from build123d import *

# Parameters (mm, degrees)
SKETCH1_R           = 3
SKETCH1_R_2         = 0.5
BOSS_EXTRUDE1_DEPTH = 5
CUT_EXTRUDE1_DEPTH  = 25
CUT_EXTRUDE2_DEPTH  = 2
SKETCH4_W           = 1
SKETCH4_H           = 3
CUT_EXTRUDE3_DEPTH  = 3


with BuildPart() as part:
    # Sketch1 → Boss-Extrude1 (new body)
    with BuildSketch(Plane.XY):
        with BuildLine():
            Line((-9.495764101, 3), (-6.495764101, 5))
            Line((-6.495764101, 5), (5.504235899, 5))
            ThreePointArc((5.504235899, 5), (9.046847958, 3.528441554), (10.504195739, -0.02004008))
            ThreePointArc((10.504195739, -0.02004008), (9.032677453, -3.542612059), (5.504235899, -5))
            Line((5.504235899, -5), (-6.495764101, -5))
            Line((-6.495764101, -5), (-9.495764101, -3))
            Line((-9.495764101, -3), (-9.495764101, 3))
        make_face()
        with Locations((-4.495764101, 0)):
            Circle(SKETCH1_R, mode=Mode.SUBTRACT)
        with Locations((-0.495764101, 0)):
            Circle(SKETCH1_R_2, mode=Mode.SUBTRACT)
        with BuildLine():
            Line((2.504235899, 2), (5.504235899, 2))
            ThreePointArc((5.504235899, 2), (7.504235899, 0), (5.504235899, -2))
            Line((5.504235899, -2), (2.504235899, -2))
            ThreePointArc((2.504235899, -2), (0.504235899, 0), (2.504235899, 2))
        make_face(mode=Mode.SUBTRACT)
    extrude(amount=BOSS_EXTRUDE1_DEPTH)

    # Sketch2 → Cut-Extrude1 (cut)
    with BuildSketch(Plane(origin=(0, 5, 0), x_dir=(1, 0, 0), z_dir=(0, 1, 0))):
        Polygon((-9.495764101, -2), (-2.495764101, -2), (-2.495764101, -3), (4.450061274, -3), (4.450061274, -5), (9.504235899, -5), (9.504235899, -3), (10.504235899, -3), (10.504235899, -6.643116644), (-9.495764101, -6.643116644), align=None)
    extrude(amount=-CUT_EXTRUDE1_DEPTH, mode=Mode.SUBTRACT)

    # Sketch3 → Cut-Extrude2 (cut)
    with BuildSketch(Plane.XY.offset(5)):
        with BuildLine():
            Line((4.450061274, 5), (4.450061274, 4))
            Line((4.450061274, 4), (5.504235899, 4))
            ThreePointArc((5.504235899, 4), (8.332663024, 2.828427125), (9.504235899, 0))
            Line((9.504235899, 0), (9.504235899, 3))
            ThreePointArc((9.504235899, 3), (7.740303877, 4.472135955), (5.504235899, 5))
            Line((5.504235899, 5), (4.450061274, 5))
        make_face()
        with BuildLine():
            Line((5.504235899, -4), (4.450061274, -4))
            Line((4.450061274, -4), (4.450061274, -5))
            Line((4.450061274, -5), (5.504235899, -5))
            ThreePointArc((5.504235899, -5), (7.740303877, -4.472135955), (9.504235899, -3))
            Line((9.504235899, -3), (9.504235899, 0))
            ThreePointArc((9.504235899, 0), (8.332663024, -2.828427125), (5.504235899, -4))
        make_face()
        with BuildLine():
            Line((4.450061274, -4), (4.450061274, -2))
            Line((4.450061274, -2), (2.504235899, -2))
            ThreePointArc((2.504235899, -2), (0.504235899, 0), (2.504235899, 2))
            Line((2.504235899, 2), (4.450061274, 2))
            Line((4.450061274, 2), (4.450061274, 4))
            Line((4.450061274, 4), (4.429293772, 4))
            Line((4.429293772, 4), (2.504235899, 4))
            ThreePointArc((2.504235899, 4), (-1.495764101, 0), (2.504235899, -4))
            Line((2.504235899, -4), (4.450061274, -4))
        make_face()
    extrude(amount=-CUT_EXTRUDE2_DEPTH, mode=Mode.SUBTRACT)

    # Sketch4 → Cut-Extrude3 (cut)
    with BuildSketch(Plane.ZY.offset(9.495764101)):
        with Locations((1.5, 0)):
            Rectangle(SKETCH4_W, SKETCH4_H)
    extrude(amount=-CUT_EXTRUDE3_DEPTH, mode=Mode.SUBTRACT)


solid = part.part
Read the model definition and answer for the solid it produces. Units are mm, in the model's axes. A direction names the side the tool comes from. Give positions to 0.01 mm unless a question says otherwise; leave off trailing zeros. Write each loop counter-clockwise with the first axis right and the second up, starting at its lowest first coordinate (ties: lowest second). Pieces come first, ordered by that corner, then holes. Notation, with made-up numbers: (-5, 67) - (14, 67) arc R27 ccw to (14, 88) - close; hole circle Ø4 at (-38.75, -3.5). An arc over 180 degrees is marked (long way). Return JSON: item names as keys, results as strings.
Q1. For faces 4 (the face through (4, 2, 2)), 5 (the face through (-8, 0, 1)), 6 (the face through (-2.496, -3.6, 2.5)), determine the directions among +Z, -Z, +X, -X, +Y, -Y from which every point of the face is accessible in a straight line to the end or side of a thin tool.
Reply:
{"face 4": "+Z, -Z", "face 5": "+Z, -X", "face 6": "+Z, -X, +Y, -Y"}
Q2. Consider line 1 along X through (y, z) = (0, 1.45); line 2 along Y through (x, z) = (3.75, 2.5); line 3 along X through (y, z) = (-1.5, 0.95). Determine where each line is inside the solid, lowest interval first. Write a range as [from, to].
Reply:
{"line 1": "[-1.5, -1], [0, 0.5], [7.5, 10.5]", "line 2": "[-5, -2], [2, 5]", "line 3": "[-9.5, -7.09], [-1.9, 1.18], [6.83, 10.27]"}
Q3. A cutting plane is placed at C-C, the plane y = -1.75. Determine the outline of the cut face in (x, z).
Reply:
{"outline": "(-9.5, 0) - (-6.93, 0) - (-6.93, 2) - (-9.5, 2) - close; (-2.06, 0) - (1.54, 0) - (1.54, 3) - (-2.06, 3) - close; (6.47, 0) - (10.19, 0) - (10.19, 3) - (9.1, 3) - (9.1, 5) - (6.47, 5) - close"}
Q4. A cutting plane is placed at D-D, the plane z = 4.25. Determine the outline of the cut face in (x, y).
Reply:
{"outline": "(4.45, -4) - (5.5, -4) arc R4 ccw to (5.5, 4) - (4.45, 4) - (4.45, 2) - (5.5, 2) arc R2 cw to (5.5, -2) - (4.45, -2) - close"}
Q5. A cutting plane is placed at B-B, the plane z = 1.35. Determine the outline of the cut face in (x, y).
Reply:
{"outline": "(-9.5, -3) - (-6.5, -5) - (5.5, -5) arc R5 ccw to (5.5, 5) - (-6.5, 5) - (-9.5, 3) - (-9.5, 1.5) - (-7.09, 1.5) arc R3 cw (long way) to (-7.09, -1.5) - (-9.5, -1.5) - close; hole circle Ø1 at (-0.5, 0); hole (2.5, -2) - (5.5, -2) arc R2 ccw to (5.5, 2) - (2.5, 2) arc R2 ccw to start"}
Q6. Given P1, Ø0.8, axis at x = 5, z = 4, coming from the +Y side; P2, Ø4, axis at x = 1.5, y = 4, coming from the +Z side; P3, Ø1, axis at y = -3.5, z = 4, coming from the -X side, each flat-ended and moving along its own axis, determine where each tip first touches the part or whether it passes through.
Reply:
{"P1": "y = 4", "P2": "z = 3", "P3": "x = 4.45"}
Q7. For a pull along Y with two mould halves and no side action, classify faces 1 (the face through (-8.017, 3.986, 0.986)), 2 (the face through (0.6, -1, 0)), 3 (the face through (-0.034, -0.192, 1.479)) as released by +Y, released by -Y, zero draft, split by the parting line, or undercut.
Reply:
{"face 1": "released by +Y", "face 2": "zero draft", "face 3": "undercut"}
Q8. A cutting plane is placed at A-A, the plane x = 3.5. Determine the outline of the cut face in (y, z), and give its area (3 significant figures).
Reply:
{"outline": "(-5, 0) - (-2, 0) - (-2, 3) - (-5, 3) - close; (2, 0) - (5, 0) - (5, 3) - (2, 3) - close", "area": "18.0 mm²"}
